Geometry: see drawing. Coordinates: mm, zero at the bounding-box minimum. A direction names the side the tool comes from. Give positions to 0.01 mm unless a question says otherwise; leave off trailing zeros. Write each loop counter-clockwise with the first axis right and the second up, starting at its lowest first coordinate (ties: lowest second). Pieces come first, ordered by that corner, then holes. Notation, with made-up numbers: M 21.25,20.5 L 25.25,20.5 A6 cw 25.25,29.5 Z; hole C 22.5,51 d1. An arc over 180 degrees is marked long. Use CSV: the item, a comma, the result in double quotes. Start each with the question number.
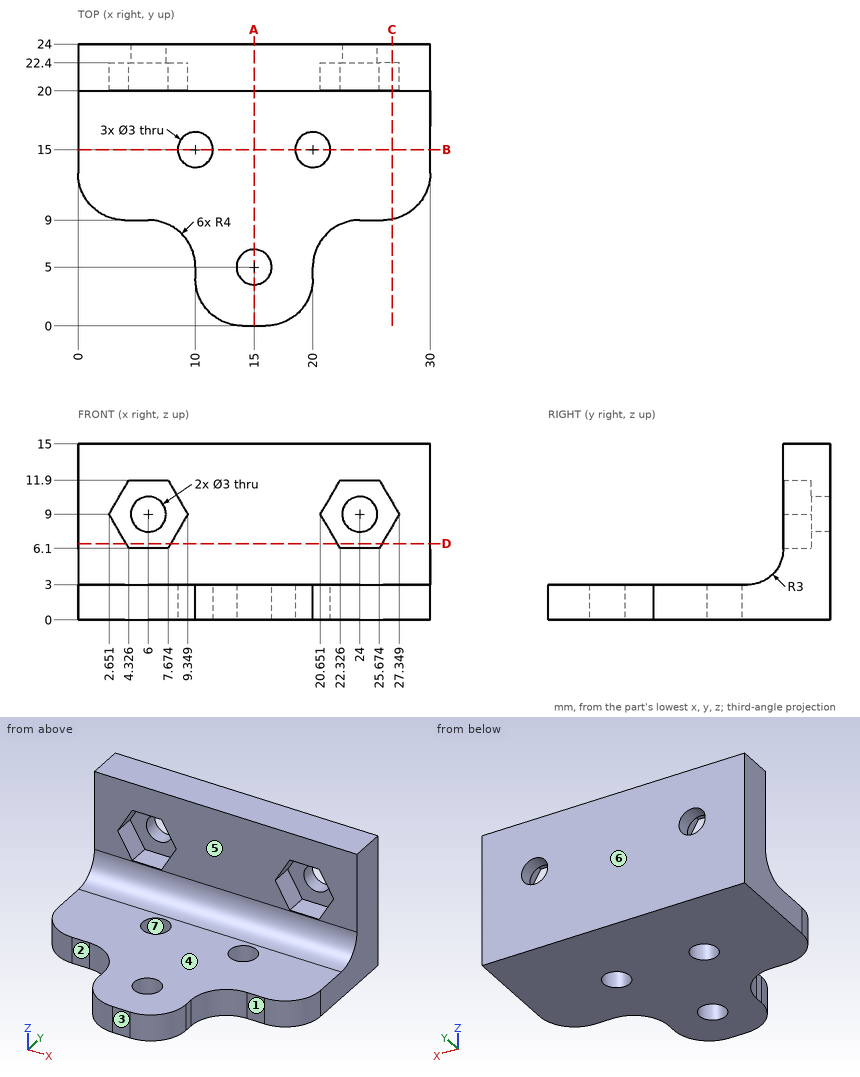
1. Section B-B on y = 15. Return loops of the section in (x, z).
2. Line query: probe 1 along Y at (x, z) = (15, 0.8); probe 2 along Y at (x, z) = (27.25, 7.25); probe 3 along Y at (x, z) = (25, 6.75). Output: solid intervals per line, ascending.
3. Section D-D on z = 6.5. Return loops of the section in (x, y) (1 decimal), then the cut area to 3 significant figures.
4. First-contact query: pin 1 (3 mm diameter, centred on x = 24, z = 7.5, fed in from -Y); pin 2 (5 mm diameter, centred on x = 10, y = 15, fed in from +Z); pin 3 (8 mm diameter, centred on x = 23.5, z = 9, fed in from -Y). Flat tips, straight axial feed; report the tip coordinate or a pass-through.
5. Access query for the marked faces 1, 2 and 3. Directions: +Z, -Z, +X, -X, +Y, -Y. A direction counts if a zero-diameter tool reaches every point of the face in a straight line with its end or side. Return the directions, or none.
6. Section C-C on x = 26.75. Return loops of the section in (y, z).
7. Pull-direction query (Y, two-part tool) for the marked faces 4, 5, 6 and 7; classes: released by +Y, released by -Y, zero draft, split by the parting line, or undercut.
8. Section A-A on x = 15. Return loops of the section in (y, z).
Resolved:
1,outline,"M 0,0 L 8.5,0 L 8.5,3 L 0,3 Z; M 11.5,0 L 18.5,0 L 18.5,3 L 11.5,3 Z; M 21.5,0 L 30,0 L 30,3 L 21.5,3 Z"
2,probe 1,"y = 0 to 3.5, 6.5 to 24"
2,probe 2,"y = 20 to 24"
2,probe 3,"y = 22.4 to 24"
3,outline,"M 0,20 L 4.1,20 L 4.1,22.4 L 7.9,22.4 L 7.9,20 L 22.1,20 L 22.1,22.4 L 25.9,22.4 L 25.9,20 L 30,20 L 30,24 L 0,24 Z"
3,area,"102 mm2"
4,pin 1,"stops at y = 20"
4,pin 2,"stops at z = 3.04"
4,pin 3,"stops at y = 19.83"
5,face 1,"+Z, -Z, +X, -Y"
5,face 2,"+Z, -Z, -X, -Y"
5,face 3,"+Z, -Z, +X, -X, -Y"
6,outline,"M 9.07,0 L 24,0 L 24,15 L 20,15 L 20,10.04 L 22.4,10.04 L 22.4,7.96 L 20,7.96 L 20,6 A3 cw 17,3 L 9.07,3 Z"
7,face 4,"zero draft"
7,face 5,"released by -Y"
7,face 6,"released by +Y"
7,face 7,"undercut"
8,outline,"M 0,0 L 3.5,0 L 3.5,3 L 0,3 Z; M 6.5,0 L 24,0 L 24,15 L 20,15 L 20,6 A3 cw 17,3 L 6.5,3 Z"
